Check sheet for the modelled part. Datum: model origin and axes. Units: mm. A direction names the side the tool comes from. Give positions to 0.01 mm unless a question says otherwise; leave off trailing zeros. Order: outer loops, then holes, each group sorted by start corner. A loop starts at its lowest first (then second) coordinate and runs counter-clockwise, first axis right, second up.
```python
from build123d import *

# Parameters (mm, degrees)
F0_W     = 76.2
F0_H     = 76.2
F1_DEPTH = 25.4
F2_R     = 12.7
F3_DEPTH = 12.7


with BuildPart() as f1:
    # F0 (on Top) → F1 (new body)
    with BuildSketch(Plane.XY):
        Rectangle(F0_W, F0_H)
    extrude(amount=F1_DEPTH)

    # F2 (on face) → F3 (join, symmetric)
    with BuildSketch(Plane.XY.offset(25.4)):
        with Locations((-38.1, 38.1)):
            Circle(F2_R)
        with Locations((38.1, 38.1)):
            Circle(F2_R)
        with Locations((-38.1, -38.1)):
            Circle(F2_R)
        with Locations((38.1, -38.1)):
            Circle(F2_R)
    extrude(amount=F3_DEPTH, both=True)


solid = f1.part
```
Q1. Sectioned sample at B-B, the plane x = -44. Record the cut outline in (y, z), plus the area to 3 significant figures.
Q2. Sectioned sample at A-A, the plane z = 30.5. Record the cut outline in (x, y).
Q3. Go/stop test with flat-tipped pins: P1, Ø5, axis at y = -24, z = 34, coming from the +X side; P2, Ø7.5, axis at x = 8, z = 13, coming from the -Y side; P3, Ø12, axis at x = 31.5, z = 10.5, coming from the +Y side; P4, Ø4, axis at x = -10, y = 8, coming from the -Z side. Record where each tip stops, or that it passes through.
Q4. Sectioned sample at D-D, the plane z = 20.5. Record the cut outline in (x, y), plus the area to 3 significant figures.
Q5. Material ranges on line 1 (Z direction, x = -7, y = 1.5); line 2 (Y direction, x = -3, z = 13.5), recorded low to high.
Q6. Sectioned sample at C-C, the plane y = -43.5. Record the cut outline in (x, z).
Q7. Draft check along X on faces 4 (the flat face through (-1, -38.1, 13)), 5 (the flat face through (-38.1, -1, 13)), 6 (the flat face through (-1, 38.1, 13)), 7 (the flat face through (-38, 38, 38.1)). Enter one of: pulls with the +X half, pulls with the -X half, needs draft (parallel to the pull), parting line crosses it, or undercut.
Q8. Tool access check on faces 1 (the flat face through (-1, 1, 0)), 2 (the flat face through (-1, 1, 25.4)), 3 (the flat face through (38.1, -1, 13)). Record the directions out of +Z, -Z, +X, -X, +Y, -Y that give a thin tool (end or side, any length) a straight path to the whole face; none if there is none.
Filled in:
1. outline: (-49.35, 12.7) - (-26.85, 12.7) - (-26.85, 38.1) - (-49.35, 38.1) - close; (26.85, 12.7) - (49.35, 12.7) - (49.35, 38.1) - (26.85, 38.1) - close
1. area: 1,140 mm2
2. outline: circle Ø25.4 at (-38.1, -38.1); circle Ø25.4 at (-38.1, 38.1); circle Ø25.4 at (38.1, -38.1); circle Ø25.4 at (38.1, 38.1)
3. P1: stops at x = 43.27
3. P2: stops at y = -38.1
3. P3: stops at y = 50.76
3. P4: stops at z = 0
4. outline: (-38.1, -25.4) arc R12.7 ccw (long way) to (-25.4, -38.1) - (25.4, -38.1) arc R12.7 ccw (long way) to (38.1, -25.4) - (38.1, 25.4) arc R12.7 ccw (long way) to (25.4, 38.1) - (-25.4, 38.1) arc R12.7 ccw (long way) to (-38.1, 25.4) - close
4. area: 7,330 mm2
5. line 1: z = 0 to 25.4
5. line 2: y = -38.1 to 38.1
6. outline: (-49.59, 12.7) - (-26.61, 12.7) - (-26.61, 38.1) - (-49.59, 38.1) - close; (26.61, 12.7) - (49.59, 12.7) - (49.59, 38.1) - (26.61, 38.1) - close
7. face 4: undercut
7. face 5: pulls with the -X half
7. face 6: undercut
7. face 7: needs draft
8. face 1: -Z, +X, -X, +Y, -Y
8. face 2: +Z
8. face 3: -Z, +X
